Read the model definition and answer for the solid it produces. Units are mm, in the model's axes. A direction names the side the tool comes from. Coordinates: 2 decimals unless noted, no trailing zeros. Loops run counter-clockwise (first coordinate to the right, second up) from the corner with the lowest first, then second, coordinate; pieces in that order, holes last. Notation, with made-up numbers: (-34, 79) - (-19, 79) arc R29 cw to (-19, 102) - close; hole circle Ø4 at (40, 39.25). An arc over 180 degrees is marked (long way). One line per item, written item: value. Start each with the question number.
from build123d import *

# Parameters (mm, degrees)
F0_W     = 45
F0_H     = 35
F1_DEPTH = 4.5
F2_W     = 15
F2_H     = 1.5
F3_DEPTH = 35.001
F4_R     = 3
F5_DEPTH = 3.5
F6_R     = 1.75
F7_DEPTH = 4.501
F8_W     = 10
F8_H     = 10
F9_DEPTH = 3
F10_SIZE = 2


with BuildPart() as f1:
    # F0 (on Front) → F1 (new body)
    with BuildSketch(Plane.XZ):
        with Locations((0, 2.5)):
            Rectangle(F0_W, F0_H)
    extrude(amount=F1_DEPTH)

    # F2 (on face) → F3 (cut, through all)
    with BuildSketch(Plane.XY.offset(20)):
        with Locations((-2.5, -2.25)):
            Rectangle(F2_W, F2_H)
    extrude(amount=-F3_DEPTH, mode=Mode.SUBTRACT)

    # F4 (on face) → F5 (cut)
    with BuildSketch(Plane.XZ.offset(4.5)):
        with Locations((17.5, -7.5)):
            Circle(F4_R)
        with Locations((-17.5, -7.5)):
            Circle(F4_R)
    extrude(amount=-F5_DEPTH, mode=Mode.SUBTRACT)

    # F6 (on face) → F7 (cut, through all)
    with BuildSketch(Plane.XZ.offset(4.5)):
        with Locations((17.5, -7.5)):
            Circle(F6_R)
        with Locations((-17.5, -7.5)):
            Circle(F6_R)
    extrude(amount=-F7_DEPTH, mode=Mode.SUBTRACT)

    # F8 (on face) → F9 (cut)
    with BuildSketch(Plane(origin=(0, 0, 0), x_dir=(-1, 0, 0), z_dir=(0, 1, 0))):
        with Locations((5, 10)):
            Rectangle(F8_W, F8_H)
    extrude(amount=-F9_DEPTH, mode=Mode.SUBTRACT)

    # F10
    f10_edges = [f1.edges().sort_by_distance(p)[0] for p in [
        (-22.5, -2.25, 20),
        (22.5, -2.25, 20),
        (22.5, -2.25, -15),
        (-22.5, -2.25, -15),
    ]]
    chamfer(f10_edges, length=F10_SIZE)


solid = f1.part
1) For faces 4 (the cylindrical face through (-19.71, -2.77, -5.47)), 5 (the flat face through (-10, -2, 3)), 6 (the flat face through (-3, -3, 3)), determine the directions among +Z, -Z, +X, -X, +Y, -Y from which every point of the face is accessible in a straight line to the end or side of a thin tool.
2) Section A-A, the plane z = -7.5 is taken. Determine the outline of the cut face in (x, y).
3) Section C-C, the plane y = -2 is taken. Determine the outline of the cut face in (x, z), and give its area (3 significant figures).
4) Section D-D, the plane z = 16.5 is taken. Determine the outline of the cut face in (x, y).
5) Flat-ended cylindrical pins translate along their axes: P1, Ø5, axis at x = 17.5, z = -7.5, coming from the -Y side; P2, Ø3, axis at x = 17.5, z = -7.5, coming from the +Y side. Find the tip coordinate at first contact, or state that the pin passes through.
6) Straight lines are drawn through the part: L1, parallel to Y at x = -8.5, z = -3; L2, parallel to Z at x = 17.5, y = -1.7; L3, parallel to X at y = -1.55, z = 8.5. For each, find the intervals that lie inside material, in ascending order.
7) Determine the mould class of faces 1 (the flat face through (-21.5, -2.2, 19)), 2 (the flat face through (19, -1, -9)), 3 (the flat face through (0, 0, 3)) for opening direction X: released by +X, released by -X, zero draft, split by the parting line, or undercut.
8) Section B-B, the plane x = 2 is taken. Determine the outline of the cut face in (y, z).
Answer below:
1. face 4: -Y
1. face 5: none
1. face 6: +Z, -Z
2. outline: (-22.5, -4.5) - (-20.5, -4.5) - (-20.5, -1) - (-19.25, -1) - (-19.25, 0) - (-22.5, 0) - close; (-15.75, -1) - (-14.5, -1) - (-14.5, -4.5) - (14.5, -4.5) - (14.5, -1) - (15.75, -1) - (15.75, 0) - (-15.75, 0) - close; (19.25, -1) - (20.5, -1) - (20.5, -4.5) - (22.5, -4.5) - (22.5, 0) - (19.25, 0) - close; hole (-10, -3) - (5, -3) - (5, -1.5) - (-10, -1.5) - close
3. outline: (-22.5, -13) - (-20.5, -15) - (-10, -15) - (-10, 20) - (-20.5, 20) - (-22.5, 18) - close; (5, -15) - (20.5, -15) - (22.5, -13) - (22.5, 18) - (20.5, 20) - (5, 20) - close; hole circle Ø6 at (-17.5, -7.5); hole circle Ø6 at (17.5, -7.5)
3. area: 985 mm2
4. outline: (-22.5, -4.5) - (22.5, -4.5) - (22.5, 0) - (-22.5, 0) - close; hole (-10, -3) - (5, -3) - (5, -1.5) - (-10, -1.5) - close
5. P1: y = -1
5. P2: through
6. L1: -4.5 to -3, -1.5 to 0
6. L2: -15 to -10.5, -4.5 to 20
6. L3: -22.5 to -10, 5 to 22.5
7. face 1: released by -X
7. face 2: undercut
7. face 3: zero draft
8. outline: (-4.5, -15) - (-3, -15) - (-3, 20) - (-4.5, 20) - close; (-1.5, -15) - (0, -15) - (0, 20) - (-1.5, 20) - close
